The model under review builds one solid part; all positions refer to its coordinate system, in mm. A direction names the side the tool comes from. Round coordinates to 2 decimals unless told otherwise and drop trailing zeros. Write each loop counter-clockwise with the first axis right and the second up, starting at its lowest first coordinate (ties: lowest second). Pieces come first, ordered by that corner, then holes. Notation, with made-up numbers: (-10.75, -14.5) - (28.25, -14.5) arc R18 ccw to (28.25, 8.5) - close; hole circle Ø11 at (43.25, 22.5). An arc over 180 degrees is marked (long way). One line per question, with ' | ' between items. Start each with the question number.
Autodesk Inventor part; units mm, degrees
ref_plane "Work Plane1" through (0, 150, 0) normal (0, 1, 0) x (-1, 0, 0)
ref_plane "YZ Plane" through (0, 0, 0) normal (1, 0, 0) x (0, 1, 0)
ref_plane "XY Plane" through (0, 0, 0) normal (0, 0, 1) x (1, 0, 0)
sketch "Sketch1" plane through (0, 0, 0) normal (0, 0, 1) x (1, 0, 0)
  line L0 (0, 0) -> (400, 0)
  line L1 (400, 0) -> (400, 300)
  line L2 (400, 300) -> (0, 300)
  line L3 (0, 300) -> (0, 0)
  dimension "d0" = 400
  dimension "d1" = 300
extrude "Extrusion1" add sketch "Sketch1" along normal blind 30
sketch "Sketch2" plane through (0, 0, 30) normal (0, 0, 1) x (1, 0, 0)
  line L0 (20, 280) -> (50, 280)
  line L1 (50, 280) -> (50, 250)
  line L2 (50, 250) -> (20, 250)
  line L3 (20, 250) -> (20, 280)
  line L4 (350, 280) -> (380, 280)
  line L5 (380, 280) -> (380, 250)
  line L6 (380, 250) -> (350, 250)
  line L7 (350, 250) -> (350, 280)
  line L8 (350, 20) -> (380, 20)
  line L9 (380, 20) -> (380, 50)
  line L10 (380, 50) -> (350, 50)
  line L11 (350, 50) -> (350, 20)
  line L12 (0, 300) -> (0, 0)
  line L13 (400, 300) -> (0, 300)
  line L14 (400, 0) -> (400, 300)
  line L15 (0, 0) -> (400, 0)
  line L16 (20, 50) -> (50, 50)
  line L17 (50, 50) -> (50, 20)
  line L18 (50, 20) -> (20, 20)
  line L19 (20, 20) -> (20, 50)
  dimension "d4" = 30
  dimension "d5" = 30
  dimension "d6" = 30
  dimension "d7" = 30
  dimension "d10" = 30
  dimension "d11" = 30
  dimension "d12" = 20
  dimension "d13" = 20
  dimension "d14" = 20
  dimension "d15" = 20
  dimension "d16" = 20
  dimension "d17" = 30
  dimension "d18" = 30
  dimension "d19" = 20
  dimension "d20" = 20
extrude "Extrusion2" add sketch "Sketch2" along normal blind 300 contours L0 L1 L2 L3 | L4 L5 L6 L7 | L11 L10 L9 L8 | L16 L17 L18 L19
sketch "Sketch3" plane through (0, 0, 0) normal (0, 0, -1) x (-1, 0, 0)
  line L0 (-400, 300) -> (0, 300)
  line L1 (0, 300) -> (-20, 300)
  line L2 (-20, 300) -> (-20, 285)
  line L3 (-20, 285) -> (0, 285)
  line L4 (0, 285) -> (0, 300)
  line L5 (0, 300) -> (0, 0)
  line L6 (-20, 20) -> (-50, 20)
  line L7 (0, 0) -> (-20, 0)
  line L8 (0, 190) -> (-20, 190)
  line L9 (-20, 190) -> (-20, 205)
  line L10 (-20, 205) -> (0, 205)
  line L11 (0, 205) -> (0, 190)
  line L12 (0, 110) -> (-20, 110)
  line L13 (-20, 110) -> (-20, 95)
  line L14 (-20, 95) -> (0, 95)
  line L15 (0, 95) -> (0, 110)
  line L16 (0, 0) -> (-20, 0)
  line L17 (-20, 0) -> (-20, 15)
  line L18 (-20, 15) -> (0, 15)
  line L19 (0, 15) -> (0, 0)
  point P0 (0, 95)
  point P1 (0, 205)
  dimension "d31" = 20
  dimension "d32" = 15
  dimension "d33" = 20
  dimension "d34" = 15
  dimension "d35" = 20
  dimension "d36" = 15
  dimension "d37" = 15
  dimension "d38" = 20
  dimension "d39" = 80
  dimension "d40" = 80
  dimension "d41" = 80
extrude "Extrusion3" add sketch "Sketch3" along normal blind 385
sketch "Sketch4" plane through (0, 0, 0) normal (0, 1, 0) x (-1, 0, 0)
  line L0 (-20, 0) -> (-20, -385)
  line L1 (0, -400) -> (-20, -400)
  line L2 (-20, -400) -> (-20, -385)
  line L3 (-20, -385) -> (0, -385)
  line L4 (0, -385) -> (0, -400)
  point P0 (0, 0)
  dimension "d44" = 20
  dimension "d45" = 15
extrude "Extrusion4" add sketch "Sketch4" along normal blind 300
sketch "Sketch5" plane through (0, 0, 0) normal (0, 1, 0) x (-1, 0, 0)
  line L0 (-20, 0) -> (-20, -385)
  line L1 (-20, -120) -> (-205, -120)
  line L2 (-205, -120) -> (-205, -100)
  line L3 (-205, -100) -> (-20, -100)
  line L4 (-20, -100) -> (-20, -120)
  line L5 (-400, 0) -> (-20, 0)
  point P0 (0, 0)
  point P1 (-20, -100)
  dimension "d48" = 185
  dimension "d49" = 20
  dimension "d50" = 100
ref_plane "Work Plane1" through (0, 150, 0) normal (0, 1, 0) x (-1, 0, 0)
extrude "Extrusion5" add sketch "Sketch5" along normal blind 20
mirror "Mirror1" about plane through (0, 150, 0) normal (0, 1, 0) of "Extrusion5"
properties part number "Maitri_chair"
1. Add section B-B, the plane x = 33. Write out the cut boundary in (y, z).
2. Add section A-A, the plane z = 245. Write out the cut boundary in (x, y), then the cut area to 3 significant figures.
3. Machinability: for faces 1 (the face through (350, 35, 178)), 2 (the face through (111, 280, -110)), 3 (the face through (20, 7, -51)), 4 (the face through (35, 250, 178)), which of the approach directions +Z, -Z, +X, -X, +Y, -Y give a long, thin tool a straight path to every point of the face, cutting with its end or side? Answer none if there is none.
4. Wall thickness on line 1 along Y through (x, z) = (35, 255); line 2 along Z through (x, y) = (133.5, 17.5); line 3 along X through (y, z) = (40, 212): over which ranges is each line inside the solid? List them lowest first. Write a range as [from, to].
5. The part is to be moulded in two halves that separate along Z. For faces 5 (the face through (111, 290, -100)), 6 (the face through (35, 265, 330)), 7 (the face through (365, 280, 178)), say which applies: pulls with the +Z half, pulls with the -Z half, needs draft (parallel to the pull), parting line crosses it, or undercut.
6. Clearance check with flat-ended pins moving along their axes: P1, Ø8, axis at y = 254, z = 209, coming from the +X side; P2, Ø10, axis at x = 138, y = 5.5, coming from the +Z side; P3, Ø3, axis at x = 254, z = -3, coming from the -Y side; P4, Ø24, axis at x = 358.5, z = 240, coming from the +Y side. State where each tip first meets the part, or that it passes through.
7. Add section D-D, the plane x = 122.5. Write out the cut boundary in (y, z), then the cut area to 3 significant figures.
8. Add section C-C, the plane y = 224. Write out the cut boundary in (x, z).
Geometry check:
1) outline: (0, -120) - (20, -120) - (20, -100) - (0, -100) - close; (0, 0) - (300, 0) - (300, 30) - (280, 30) - (280, 330) - (250, 330) - (250, 30) - (50, 30) - (50, 330) - (20, 330) - (20, 30) - (0, 30) - close; (280, -120) - (300, -120) - (300, -100) - (280, -100) - close
2) outline: (20, 20) - (50, 20) - (50, 50) - (20, 50) - close; (20, 250) - (50, 250) - (50, 280) - (20, 280) - close; (350, 20) - (380, 20) - (380, 50) - (350, 50) - close; (350, 250) - (380, 250) - (380, 280) - (350, 280) - close | area: 3,600 mm2
3) face 1: +Z, +Y, -Y | face 2: -Z, +X, -X | face 3: +X, +Y, -Y | face 4: +Z, +X, -X
4) line 1: y = [20, 50], [250, 280] | line 2: z = [-120, -100], [0, 30] | line 3: x = [20, 50], [350, 380]
5) face 5: undercut | face 6: pulls with the +Z half | face 7: needs draft
6) P1: stops at x = 380 | P2: stops at z = 30 | P3: passes through | P4: stops at y = 280
7) outline: (0, -120) - (20, -120) - (20, -100) - (0, -100) - close; (0, 0) - (300, 0) - (300, 30) - (0, 30) - close; (280, -120) - (300, -120) - (300, -100) - (280, -100) - close | area: 9,800 mm2
8) outline: (0, -400) - (20, -400) - (20, -385) - (0, -385) - close; (0, 0) - (400, 0) - (400, 30) - (0, 30) - close
